from build123d import *

# Parameters (mm, degrees)
SKETCH1_W                                           = 60
SKETCH1_H                                           = 35
BOSS_EXTRUDE1_DEPTH                                 = 3
CSK_FOR_M3_COUNTERSUNK_FLAT_HEAD_SCREW1_D           = 3.4
CSK_FOR_M3_COUNTERSUNK_FLAT_HEAD_SCREW1_DEPTH       = 3
CSK_FOR_M3_COUNTERSUNK_FLAT_HEAD_SCREW1_CSINK_D     = 6.3
CSK_FOR_M3_COUNTERSUNK_FLAT_HEAD_SCREW1_CSINK_ANGLE = 90
CSK_FOR_M3_COUNTERSUNK_FLAT_HEAD_SCREW1_TIP         = 1.021463052
BOSS_EXTRUDE2_DEPTH                                 = 15
BOSS_EXTRUDE3_DEPTH                                 = 15
CUT_EXTRUDE4_DEPTH                                  = 15
SKETCH8_W                                           = 3
SKETCH8_H                                           = 6
CUT_EXTRUDE5_DEPTH                                  = 15
FILLET4_R                                           = 1.5


with BuildPart() as part:
    # Sketch1 → Boss-Extrude1 (new body)
    with BuildSketch(Plane.XY):
        Rectangle(SKETCH1_W, SKETCH1_H)
    extrude(amount=BOSS_EXTRUDE1_DEPTH)

    # CSK for M3 Countersunk Flat Head Screw1
    with Locations(Plane(origin=(0, 0, 0), x_dir=(1, 0, 0), z_dir=(0, 0, -1))):
        with Locations((0, -4.5), (-15, 9.5), (15, 9.5)):
            CounterSinkHole(CSK_FOR_M3_COUNTERSUNK_FLAT_HEAD_SCREW1_D / 2, CSK_FOR_M3_COUNTERSUNK_FLAT_HEAD_SCREW1_CSINK_D / 2, depth=CSK_FOR_M3_COUNTERSUNK_FLAT_HEAD_SCREW1_DEPTH, counter_sink_angle=CSK_FOR_M3_COUNTERSUNK_FLAT_HEAD_SCREW1_CSINK_ANGLE)
            with Locations((0, 0, -(CSK_FOR_M3_COUNTERSUNK_FLAT_HEAD_SCREW1_DEPTH + CSK_FOR_M3_COUNTERSUNK_FLAT_HEAD_SCREW1_TIP / 2))):  # 118° drill point
                Cone(0, CSK_FOR_M3_COUNTERSUNK_FLAT_HEAD_SCREW1_D / 2, CSK_FOR_M3_COUNTERSUNK_FLAT_HEAD_SCREW1_TIP, mode=Mode.SUBTRACT)

    # Sketch5 → Boss-Extrude2 (add)
    with BuildSketch(Plane(origin=(30, 0, 0), x_dir=(0, 0, -1), z_dir=(1, 0, 0))):
        with BuildLine():
            Line((-5.479055467, 14.545576741), (-4.958110934, 11.591153482))
            ThreePointArc((-4.958110934, 11.591153482), (-8.05212086, 23.138155725), (-3, 12.303847577))
            Line((-3, 12.303847577), (-3, 17.5))
            ThreePointArc((-3, 17.5), (-8.298133329, 19.428362829), (-5.479055467, 14.545576741))
        make_face()
    extrude(amount=-BOSS_EXTRUDE2_DEPTH)

    # Sketch6 → Boss-Extrude3 (add)
    with BuildSketch(Plane.ZY):
        with BuildLine():
            Line((3, 12.335251693), (3, 17.5))
            ThreePointArc((3, 17.5), (8.298133329, 19.428362829), (5.479055467, 14.545576741))
            Line((5.479055467, 14.545576741), (4.962830018, 11.617916738))
            ThreePointArc((4.962830018, 11.617916738), (8.050201874, 23.109928462), (3, 12.335251693))
        make_face()
    extrude(amount=BOSS_EXTRUDE3_DEPTH)

    # Sketch9 → Cut-Extrude4 (cut)
    with BuildSketch(Plane.ZY.offset(15)):
        Polygon((0.004777877, 17.5), (0, 17.5), (0, 11.5), (3, 11.5), (3, 17.5), (0.027176122, 17.5), align=None)
    extrude(amount=CUT_EXTRUDE4_DEPTH, mode=Mode.SUBTRACT)

    # Sketch8 → Cut-Extrude5 (cut)
    with BuildSketch(Plane(origin=(0, 0, 0), x_dir=(0, 0, -1), z_dir=(1, 0, 0))):
        with Locations((-1.5, 14.5)):
            Rectangle(SKETCH8_W, SKETCH8_H)
    extrude(amount=CUT_EXTRUDE5_DEPTH, mode=Mode.SUBTRACT)

    # Fillet4
    fillet4_edges = [part.edges().sort_by_distance(p)[0] for p in [
        (-22.5, 11.5, 0),
        (-22.5, 11.5, 3),
        (7.5, 11.5, 0),
        (7.5, 11.5, 3),
    ]]
    fillet(fillet4_edges, radius=FILLET4_R - 0.0001)  # a hair under: the kernel refuses the full size


solid = part.part
Source: CAD feature listing. Evaluate the final solid. Frame: model axes, mm. A direction names the side the tool comes from. Round coordinates to 2 decimals unless told otherwise and drop trailing zeros. Loops run counter-clockwise (first coordinate to the right, second up) from the corner with the lowest first, then second, coordinate; pieces in that order, holes last. Notation, with made-up numbers: M 69,-9.75 L 123,-9.75 A20 ccw 123,1.25 Z; hole C 61.5,-2.75 d4. An arc over 180 degrees is marked long. Answer as CSV lines item,"result".
Q1. Line query: line 1 along X through (y, z) = (17.5, 2.75); line 2 along Y through (x, z) = (-7.5, 6); line 3 along Z through (x, y) = (7.5, 4). Output: solid intervals per line, ascending.
Verdict:
line 1,"x = -15 to 0, 15 to 30"
line 2,"y = 11.53 to 14.5, 20.5 to 23.47"
line 3,"z = 0 to 3"
Q2. Reachability of faces 4 (the face through (-7.395, 13.102, 5.225)), 5 (the face through (7.6, 11.07, 0.45)), 6 (the face through (-22.6, 11.05, 2.57)) from +Z, -Z, +X, -X, +Y, -Y: full face, straight path, thin tool, end or side. Return the list, or none.
Verdict:
face 4,"+X, -X"
face 5,"-Z, +Y"
face 6,"+Z, -X, +Y"
Q3. Cut plane D-D (y = 19.5). Return the cut outline in (x, z).
Verdict:
outline,"M -15,0.37 L 0,0.37 L 0,3.76 L -15,3.76 Z; M -15,8.24 L 0,8.24 L 0,11.63 L -15,11.63 Z; M 15,0.34 L 30,0.34 L 30,3.76 L 15,3.76 Z; M 15,8.24 L 30,8.24 L 30,11.66 L 15,11.66 Z"
Q4. Pull-direction query (Z, two-part tool) for faces 1 (the face through (-22.6, 11.07, 0.45)), 2 (the face through (22.605, 19.506, 8.231)), 3 (the face through (-15, 20, 3)); classes: +Z half, -Z half, draft (parallel to the pull), parting line (faces both ways), or undercut.
Verdict:
face 1,"-Z half"
face 2,"undercut"
face 3,"draft"
Q5. Contact query for flat-ended pins moving along their axis: pin 1 (4 mm diameter, centred on x = -0.5, z = 10.5, fed in from -Y); pin 2 (7 mm diameter, centred on y = 17.5, z = 6, fed in from -X); pin 3 (5.5 mm diameter, centred on x = -15, y = -9.5, fed in from -Z). Output: stop coordinate, or through.
Verdict:
pin 1,"stops at y = 12.08"
pin 2,"stops at x = -15"
pin 3,"stops at z = 0.4"
Q6. Cut plane A-A (y = -9.5). Return the cut outline in (x, z).
Verdict:
outline,"M -30,0 L -18.15,0 L -16.7,1.45 L -16.7,3 L -30,3 Z; M -13.3,1.45 L -11.85,0 L 11.85,0 L 13.3,1.45 L 13.3,3 L -13.3,3 Z; M 16.7,1.45 L 18.15,0 L 30,0 L 30,3 L 16.7,3 Z"
Q7. Cut plane B-B (z = 4.25). Return the cut outline in (x, y).
Verdict:
outline,"M -15,19.94 L 0,19.94 L 0,23.21 L -15,23.21 Z; M 15,19.94 L 30,19.94 L 30,23.24 L 15,23.24 Z"
